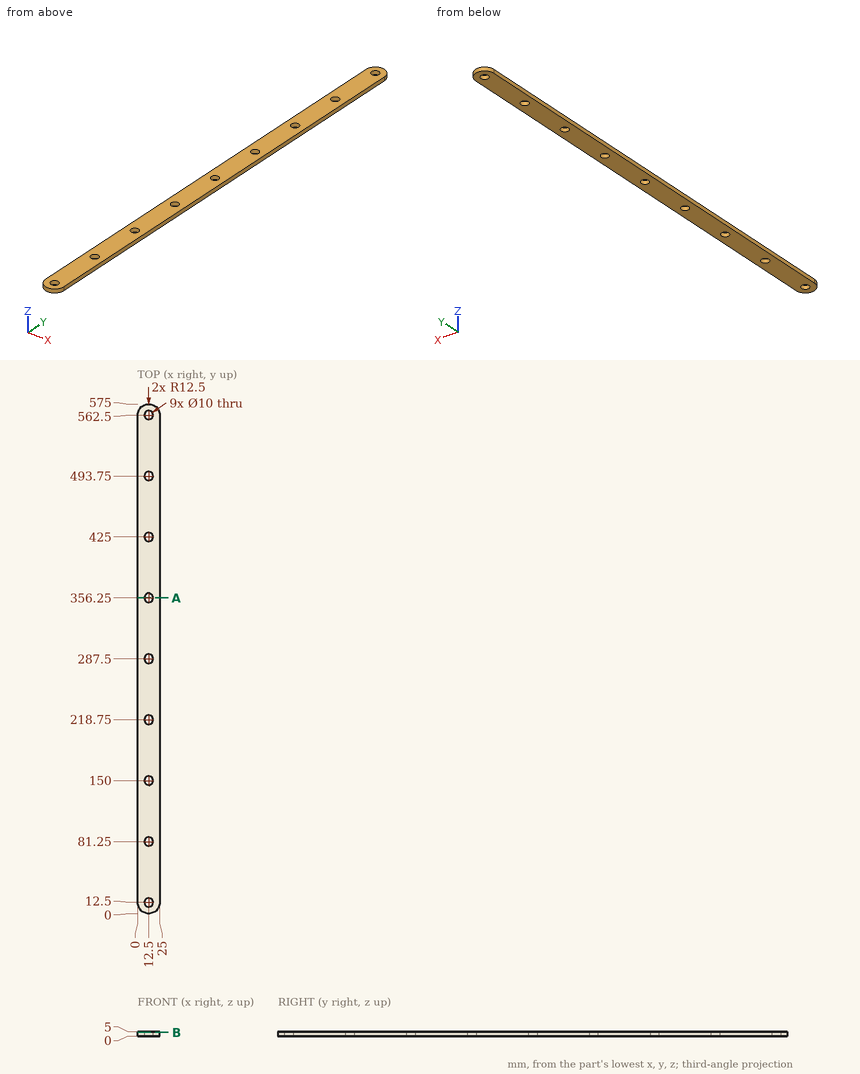
Geometry check sheet. Reference: drawing and pictorial views, mm from the part's lowest x, y, z. Coordinates: 2 decimals unless noted, no trailing zeros. Order: outer loops, then holes, each group sorted by start corner. A loop starts at its lowest first (then second) coordinate and runs counter-clockwise, first axis right, second up.
1. Go/stop test with flat-tipped pins: pin 1 Ø1.5 at (x, z) = (9, 4) entering from +Y; pin 2 Ø2 at (x, z) = (14.5, 3) entering from -Y; pin 3 Ø9 at (x, y) = (12.5, 493.75) entering from -Z. Record where each tip stops, or that it passes through.
Results found:
pin 1: stops at y = 574.69
pin 2: stops at y = 0.04
pin 3: passes through
2. Sectioned sample at B-B, the plane z = 4.1. Give the number of separate pieces and of enclosed holes in the cut face, and give its area (3 significant figures).
Results found:
separate pieces: 1
enclosed holes: 9
area: 13,500 mm2
3. Scan lines: line 1 (X direction, y = 562.5, z = 3.55); line 2 (X direction, y = 153, z = 0.6); line 3 (Y direction, x = 6, z = 3.65). Record each from-to range of solid material in increasing order.
Results found:
line 1: x = 0 to 7.5, 17.5 to 25
line 2: x = 0 to 8.5, 16.5 to 25
line 3: y = 1.82 to 573.18
4. Sectioned sample at A-A, the plane y = 356.25. Record the cut outline in (x, z), and give its area (3 significant figures).
Results found:
outline: (0, 0) - (7.5, 0) - (7.5, 5) - (0, 5) - close; (17.5, 0) - (25, 0) - (25, 5) - (17.5, 5) - close
area: 75.0 mm2
